Source: CAD feature listing. Evaluate the final solid. Frame: model axes, mm. A direction names the side the tool comes from. Round coordinates to 2 decimals unless told otherwise and drop trailing zeros. Write each loop counter-clockwise with the first axis right and the second up, starting at its lowest first coordinate (ties: lowest second). Pieces come first, ordered by that corner, then holes. Notation, with made-up numbers: M -16.75,40.25 L -3.75,40.25 A20 cw -3.75,79.25 Z; hole C 59,82 d8. An arc over 180 degrees is marked long. Use a Markdown table: item, result.
```python
from build123d import *

# Parameters (mm, degrees)
SKETCH_W        = 90
SKETCH_H        = 60
SKETCH_R        = 3.25
PAD_DEPTH       = 11
SKETCH001_R     = 6.1
POCKET_DEPTH    = 4
POCKET001_DEPTH = 5.25


with BuildPart() as part:
    # Sketch → Pad (new body)
    with BuildSketch(Plane.XY):
        with Locations((45, 30)):
            Rectangle(SKETCH_W, SKETCH_H)
        with Locations((10, 40)):
            Circle(SKETCH_R, mode=Mode.SUBTRACT)
        with Locations((80, 40)):
            Circle(SKETCH_R, mode=Mode.SUBTRACT)
        with Locations((10, 20)):
            Circle(SKETCH_R, mode=Mode.SUBTRACT)
        with Locations((80, 20)):
            Circle(SKETCH_R, mode=Mode.SUBTRACT)
        with Locations((15, 50)):
            Circle(SKETCH_R, mode=Mode.SUBTRACT)
        with Locations((75, 50)):
            Circle(SKETCH_R, mode=Mode.SUBTRACT)
        with Locations((75, 10)):
            Circle(SKETCH_R, mode=Mode.SUBTRACT)
        with Locations((15, 10)):
            Circle(SKETCH_R, mode=Mode.SUBTRACT)
    extrude(amount=PAD_DEPTH)

    # Sketch001 (on Face14 of Pad) → Pocket (cut)
    with BuildSketch(Plane.XY.offset(11)):
        with Locations((15, 50)):
            Circle(SKETCH001_R)
        with Locations((75, 50)):
            Circle(SKETCH001_R)
        with Locations((75, 10)):
            Circle(SKETCH001_R)
        with Locations((15, 10)):
            Circle(SKETCH001_R)
    extrude(amount=-POCKET_DEPTH, mode=Mode.SUBTRACT)

    # Sketch002 (on Face4 of Pocket) → Pocket001 (cut)
    with BuildSketch(Plane(origin=(0, 0, 0), x_dir=(1, 0, 0), z_dir=(0, 0, -1))):
        Polygon((15.1, -17.055514), (10, -14.111027), (4.9, -17.055514), (4.9, -22.944486), (10, -25.888973), (15.1, -22.944486), align=None)
        Polygon((80, -14.111027), (74.9, -17.055514), (74.9, -22.944486), (80, -25.888973), (85.1, -22.944486), (85.1, -17.055514), align=None)
        Polygon((10, -34.111027), (4.9, -37.055514), (4.9, -42.944486), (10, -45.888973), (15.1, -42.944486), (15.1, -37.055514), align=None)
        Polygon((80, -34.111027), (74.9, -37.055514), (74.9, -42.944486), (80, -45.888973), (85.1, -42.944486), (85.1, -37.055514), align=None)
    extrude(amount=-POCKET001_DEPTH, mode=Mode.SUBTRACT)


solid = part.part
```
Q1. Section C-C on x = 70. Return loops of the section in (y, z), plus the area to 3 significant figures.
Results are:
| item | result |
|---|---|
| outline | M 0,0 L 60,0 L 60,11 L 53.49,11 L 53.49,7 L 46.51,7 L 46.51,11 L 13.49,11 L 13.49,7 L 6.51,7 L 6.51,11 L 0,11 Z |
| area | 604 mm^2 |
Q2. Section A-A on y = 40. Return loops of the section in (x, z), plus the area to 3 significant figures.
Results are:
| item | result |
|---|---|
| outline | M 0,0 L 4.9,0 L 4.9,5.25 L 6.75,5.25 L 6.75,11 L 0,11 Z; M 13.25,5.25 L 15.1,5.25 L 15.1,0 L 74.9,0 L 74.9,5.25 L 76.75,5.25 L 76.75,11 L 13.25,11 Z; M 83.25,5.25 L 85.1,5.25 L 85.1,0 L 90,0 L 90,11 L 83.25,11 Z |
| area | 808 mm^2 |
Q3. Section D-D on y = 25. Return loops of the section in (x, z).
Results are:
| item | result |
|---|---|
| outline | M 0,0 L 8.46,0 L 8.46,5.25 L 11.54,5.25 L 11.54,0 L 78.46,0 L 78.46,5.25 L 81.54,5.25 L 81.54,0 L 90,0 L 90,11 L 0,11 Z |
Q4. Mould query, pull axis X, two halves, no side actions, for faces 4 (the cylindrical face through (10.16, 46.29, 9.03)), 5 (the flat face through (0, 30, 5)), 6 (the flat face through (44, 0, 5)). Classes: +X half, -X half, draft (parallel to the pull), parting line (faces both ways), or undercut.
Results are:
| item | result |
|---|---|
| face 4 | undercut |
| face 5 | -X half |
| face 6 | draft |
Q5. Section B-B on y = 50. Return loops of the section in (x, z).
Results are:
| item | result |
|---|---|
| outline | M 0,0 L 11.75,0 L 11.75,7 L 8.9,7 L 8.9,11 L 0,11 Z; M 18.25,0 L 71.75,0 L 71.75,7 L 68.9,7 L 68.9,11 L 21.1,11 L 21.1,7 L 18.25,7 Z; M 78.25,0 L 90,0 L 90,11 L 81.1,11 L 81.1,7 L 78.25,7 Z |
Q6. First-contact query: pin 1 Ø8.5 at (x, y) = (10, 20) entering from -Z; pin 2 Ø8.5 at (x, y) = (75, 10) entering from +Z. Flat tips, straight axial feed; report the tip coordinate or a pass-through.
Results are:
| item | result |
|---|---|
| pin 1 | z = 5.25 |
| pin 2 | z = 7 |
Q7. Reachability of faces 1 (the flat face through (12.51, 24.44, 2.59)), 2 (the cylindrical face through (71.753, 10.143, 3.451)), 3 (the flat face through (18, 7, 7)) from +Z, -Z, +X, -X, +Y, -Y: full face, straight path, thin tool, end or side. Return the list, or none.
Results are:
| item | result |
|---|---|
| face 1 | -Z |
| face 2 | +Z, -Z |
| face 3 | +Z |
Q8. Line query: L1, parallel to X at y = 50, z = 1.5; L2, parallel to Y at x = 75, z = 9.8; L3, parallel to X at y = 49.5, z = 8.5. Output: solid intervals per line, ascending.
Results are:
| item | result |
|---|---|
| L1 | 0 to 11.75, 18.25 to 71.75, 78.25 to 90 |
| L2 | 0 to 3.9, 16.1 to 43.9, 56.1 to 60 |
| L3 | 0 to 8.92, 21.08 to 68.92, 81.08 to 90 |
